Can you work these out from the model? Positions are in its coordinate system, mm. A direction names the side the tool comes from. Round coordinates to 2 decimals unless told otherwise and drop trailing zeros. Write each loop counter-clockwise with the first axis right and the second up, starting at its lowest first coordinate (ties: lowest second). Pieces come first, ordered by that corner, then holes.
Q1. If we section it at A-A (z = 36): Please give me the cut outline in (x, y).
Q2. Please list where these lines run through material, in increasing order: line 1 along X through (y, z) = (-21.75, 29); line 2 along Z through (x, y) = (-36.5, -12.5); line 3 along X through (y, z) = (-9.75, 63.5).
Q3. I'm going to push flat-ended pins straight in: pin 1 Ø4 at (x, y) = (-10.5, -9) entering from -Z; pin 2 Ø7.5 at (x, y) = (-41.5, -8.5) entering from +Z; pin 3 Ø10 at (x, y) = (-10.5, -9.5) entering from +Z. Where does each tip first touch, or does it pass through?
Q4. If we section it at B-B (y = -3.75): Please give me the cut outline in (x, z), plus the area to 3 significant figures.
Q5. For faces 1 (the flat face through (-40, -13, 50.8)), 2 (the flat face through (25.4, -13, 38)), 3 (the flat face through (-26.639, -13, 38)), which set-ups out of +Z, -Z, +X, -X, +Y, -Y let a thin tool reach every point of the face, with its end or its side?
Q6. If we section it at C-C (x = -46): Please give me the cut outline in (y, z).
Q7. We'd pull the mould along X, two halves only. Please class faces 4 (the flat face through (13, -13, 76.2)), 5 (the flat face through (-52.039, -13, 26)), 6 (the flat face through (-14, -13, 25.4)), 7 (the flat face through (0, -13, 51)): +X half, -X half, draft (parallel to the pull), parting line (faces both ways), or undercut.
Q8. If we section it at D-D (z = 56.5): Please give me the cut outline in (x, y).
from build123d import *

# Parameters (mm, degrees)
F0_W     = 25.4
F0_H     = 25.4
F0_W_2   = 26.6390249144
F2_DEPTH = 25.4


with BuildPart() as f2:
    # F0 (on Front) → F2 (new body)
    with BuildSketch(Plane.XZ):
        with Locations((-39.3390249144, 38.1)):
            Rectangle(F0_W, F0_H)
        with Locations((-39.3390249144, 12.7)):
            Rectangle(F0_W, F0_H)
        with Locations((-13.3195124572, 12.7)):
            Rectangle(F0_W_2, F0_H)
        with Locations((12.7, 63.5)):
            Rectangle(F0_W, F0_H)
        with Locations((12.7, 38.1)):
            Rectangle(F0_W, F0_H)
        with Locations((12.7, 12.7)):
            Rectangle(F0_W, F0_H)
    extrude(amount=F2_DEPTH)


solid = f2.part
A:
1. outline: (-52.04, -25.4) - (-26.64, -25.4) - (-26.64, 0) - (-52.04, 0) - close; (0, -25.4) - (25.4, -25.4) - (25.4, 0) - (0, 0) - close
2. line 1: x = -52.04 to -26.64, 0 to 25.4
2. line 2: z = 0 to 50.8
2. line 3: x = 0 to 25.4
3. pin 1: stops at z = 0
3. pin 2: stops at z = 50.8
3. pin 3: stops at z = 25.4
4. outline: (-52.04, 0) - (25.4, 0) - (25.4, 76.2) - (0, 76.2) - (0, 25.4) - (-26.64, 25.4) - (-26.64, 50.8) - (-52.04, 50.8) - close
4. area: 3,900 mm2
5. face 1: +Z, -X, +Y, -Y
5. face 2: +Z, -Z, +X, +Y, -Y
5. face 3: +Z, +Y, -Y
6. outline: (-25.4, 0) - (0, 0) - (0, 50.8) - (-25.4, 50.8) - close
7. face 4: draft
7. face 5: -X half
7. face 6: undercut
7. face 7: undercut
8. outline: (0, -25.4) - (25.4, -25.4) - (25.4, 0) - (0, 0) - close
